from build123d import *

# Parameters (mm, degrees)
F0_R      = 7.9375
F1_DEPTH  = 28.575
F3_DEPTH  = 0.8128
F2_R      = 7.9375
F4_DEPTH  = 4.7752
F6_DEPTH  = 22.225
F8_DEPTH  = 25.4
F10_DEPTH = 25.4
F11_R     = 6.35


with BuildPart() as f1:
    # F0 (on Top) → F1 (new body)
    with BuildSketch(Plane.XY):
        with BuildLine():
            ThreePointArc((-9.525, 0), (0, 9.525), (9.525, 0))
            Line((9.525, 0), (9.525, -21.203784))
            Line((9.525, -21.203784), (19.05, -21.203784))
            Line((19.05, -21.203784), (19.05, 30.1752))
            Line((19.05, 30.1752), (9.767071, 45.471216))
            Line((9.767071, 45.471216), (-9.767071, 45.471216))
            Line((-9.767071, 45.471216), (-19.05, 30.1752))
            Line((-19.05, 30.1752), (-19.05, -21.203784))
            Line((-19.05, -21.203784), (-9.525, -21.203784))
            Line((-9.525, -21.203784), (-9.525, 0))
        make_face()
        with Locations((0, 30.1752)):
            Circle(F0_R, mode=Mode.SUBTRACT)
    extrude(amount=F1_DEPTH)

    # F2 (on face) → F3 (cut)
    with BuildSketch(Plane(origin=(0, 0, 0), x_dir=(1, 0, 0), z_dir=(0, 0, -1))):
        with BuildLine():
            Line((-12.7, 21.203784), (-12.7, 0))
            ThreePointArc((-12.7, 0), (0, -12.7), (12.7, 0))
            Line((12.7, 0), (12.7, 21.203784))
            Line((12.7, 21.203784), (9.525, 21.203784))
            Line((9.525, 21.203784), (9.525, 0))
            ThreePointArc((9.525, 0), (0, -9.525), (-9.525, 0))
            Line((-9.525, 0), (-9.525, 21.203784))
            Line((-9.525, 21.203784), (-12.7, 21.203784))
        make_face()
    extrude(amount=-F3_DEPTH, mode=Mode.SUBTRACT)

    # F2 (on face) → F4 (cut)
    with BuildSketch(Plane(origin=(0, 0, 0), x_dir=(1, 0, 0), z_dir=(0, 0, -1))):
        Polygon((19.05, -16.896216), (-19.05, -16.896216), (-19.05, -30.1752), (-9.767071, -45.471216), (9.767071, -45.471216), (19.05, -30.1752), align=None)
        with Locations((0, -30.1752)):
            Circle(F2_R, mode=Mode.SUBTRACT)
    extrude(amount=-F4_DEPTH, mode=Mode.SUBTRACT)

    # F5 (on face) → F6 (cut)
    with BuildSketch(Plane.XY.offset(28.575)):
        with BuildLine():
            Line((-14.808481, 19.019462), (-14.808481, 0))
            Line((-14.808481, 0), (-19.05, 0))
            Line((-19.05, 0), (-19.05, -21.203784))
            Line((-19.05, -21.203784), (-9.525, -21.203784))
            Line((-9.525, -21.203784), (-9.525, 0))
            ThreePointArc((-9.525, 0), (0, 9.525), (9.525, 0))
            Line((9.525, 0), (9.525, -21.203784))
            Line((9.525, -21.203784), (19.05, -21.203784))
            Line((19.05, -21.203784), (19.05, 0))
            Line((19.05, 0), (14.808481, 0))
            Line((14.808481, 0), (14.808481, 19.019462))
            Line((14.808481, 19.019462), (-14.808481, 19.019462))
        make_face()
    extrude(amount=-F6_DEPTH, mode=Mode.SUBTRACT)

    # F7 (on face) → F8 (cut)
    with BuildSketch(Plane.YZ.offset(19.05)):
        Polygon((0, 28.575), (0, 6.35), (18.815449, 28.575), align=None)
    extrude(amount=-F8_DEPTH, mode=Mode.SUBTRACT)

    # F9 (on face) → F10 (cut)
    with BuildSketch(Plane(origin=(-19.05, 0, 0), x_dir=(0, -1, 0), z_dir=(-1, 0, 0))):
        Polygon((-18.669238, 28.575), (0, 6.35), (0, 28.575), align=None)
    extrude(amount=-F10_DEPTH, mode=Mode.SUBTRACT)

    # F11
    f11_edges = [f1.edges().sort_by_distance(p)[0] for p in [
        (-14.808481, 19.019462, 17.4625),
        (14.808481, 19.019462, 17.4625),
    ]]
    fillet(f11_edges, radius=F11_R)


solid = f1.part
The listing builds one solid part. Answer for the finished solid, in the listing's coordinates (mm). A direction names the side the tool comes from. Give positions to 0.01 mm unless a question says otherwise; leave off trailing zeros. Write each loop counter-clockwise with the first axis right and the second up, starting at its lowest first coordinate (ties: lowest second). Pieces come first, ordered by that corner, then holes. Notation, with made-up numbers: (81, -16) - (134, -16) arc R30 cw to (134, 7) - close; hole circle Ø3 at (85, -20). An arc over 180 degrees is marked (long way). Use a Markdown table: item, result.
1. Each of these flat-tipped pins is pushed along its axis until it touches: P1, Ø1.5, axis at y = 25.5, z = 3.5, coming from the -X side; P2, Ø1.5, axis at x = -0.5, z = 6.5, coming from the -Y side; P3, Ø14.5, axis at x = -3, y = 30.5, coming from the -Z side; P4, Ø8.5, axis at x = -2.5, z = 18.5, coming from the -Y side. Where does it stop, or does it pass through?
Values follow:
| item | result |
|---|---|
| P1 | passes through |
| P2 | stops at y = 9.44 |
| P3 | stops at z = 4.78 |
| P4 | stops at y = 19.02 |
2. Find the intervals of material crossed by probe 1 along X at (y, z) = (5.5, 9.5); probe 2 along Y at (x, z) = (0, 20.5); probe 3 along Z at (x, y) = (15, 29.5) (3 decimals), in increasing order. Write a range as from..to.
Values follow:
| item | result |
|---|---|
| probe 1 | x = -19.05..-14.81, 14.81..19.05 |
| probe 2 | y = 19.02..22.24, 38.11..45.47 |
| probe 3 | z = 4.775..28.575 |
3. For a pull along X with two mould halves and no side action, classify faces 1 (the flat face through (9.525, -10, 4)), 2 (the flat face through (14.47, 37.72, 16.51)), 3 (the flat face through (-16.745, 9.465, 17.618)) as released by +X, released by -X, zero draft, split by the parting line, or undercut.
Values follow:
| item | result |
|---|---|
| face 1 | undercut |
| face 2 | released by +X |
| face 3 | zero draft |
4. Section C-C on z = 2.75 is taken. Write down the section's boundary in (x, y) (3 decimals).
Values follow:
| item | result |
|---|---|
| outline | (-19.05, -21.204) - (-9.525, -21.204) - (-9.525, 0) arc R9.525 cw to (9.525, 0) - (9.525, -21.204) - (19.05, -21.204) - (19.05, 16.896) - (-19.05, 16.896) - close |
5. Section D-D on x = -16 is taken. Write down the section's boundary in (y, z) (3 decimals).
Values follow:
| item | result |
|---|---|
| outline | (-21.204, 0) - (16.896, 0) - (16.896, 4.775) - (35.201, 4.775) - (35.201, 28.575) - (18.669, 28.575) - (0, 6.35) - (-21.204, 6.35) - close |
6. Section B-B on y = -4 is taken. Write down the section's boundary in (x, z) (3 decimals).
Values follow:
| item | result |
|---|---|
| outline | (-19.05, 0) - (-12.7, 0) - (-12.7, 0.813) - (-9.525, 0.813) - (-9.525, 6.35) - (-19.05, 6.35) - close; (9.525, 0.813) - (12.7, 0.813) - (12.7, 0) - (19.05, 0) - (19.05, 6.35) - (9.525, 6.35) - close |
7. Section A-A on x = 0 is taken. Write down the section's boundary in (y, z) (3 decimals).
Values follow:
| item | result |
|---|---|
| outline | (9.525, 0.813) - (12.7, 0.813) - (12.7, 0) - (16.896, 0) - (16.896, 4.775) - (22.238, 4.775) - (22.238, 28.575) - (19.019, 28.575) - (19.019, 6.35) - (9.525, 6.35) - close; (38.113, 4.775) - (45.471, 4.775) - (45.471, 28.575) - (38.113, 28.575) - close |
8. A tool of negligible diameter and unlimited length cuts with its end or side. For faces 4 (the flat face through (-14.808, 9, 11)), 5 (the flat face through (16.61, 9.28, 17.31)), 6 (the flat face through (0, 21, 4.775)), 7 (the flat face through (-10, -2, 0.813)), 8 (the flat face through (-9.525, -11, 4)), from which of +Z, -Z, +X, -X, +Y, -Y can it reach the whole face along a straight path? Write none if from no direction.
Values follow:
| item | result |
|---|---|
| face 4 | +Z, -Y |
| face 5 | +Z, +X, -Y |
| face 6 | -Z, +X, -X, +Y |
| face 7 | -Z, -Y |
| face 8 | +Z, -Z, -Y |
